Here's how the part is built. I have some questions about the finished solid (model axes, mm). Face numbers are marked on the shaded views. A direction names the side the tool comes from. Round coordinates to 2 decimals unless told otherwise and drop trailing zeros. Order: outer loops, then holes, each group sorted by start corner. A loop starts at its lowest first (then second) coordinate and runs counter-clockwise, first axis right, second up. Notation, with made-up numbers: (-25.75, -36) -> (-8.75, -36) arc R11 ccw to (-8.75, -18) -> close; hole circle Ø5 at (34, -5.5). An arc over 180 degrees is marked (long way). One line per item, written item: value.
```python
from build123d import *

# Parameters (mm, degrees)
F0_W     = 15
F0_H     = 20
F1_DEPTH = 17
F2_R     = 1.75
F3_DEPTH = 17.001
F2_W     = 15
F2_H     = 15
F4_DEPTH = 10
F5_R     = 1


with BuildPart() as f1:
    # F0 (on Top) → F1 (new body)
    with BuildSketch(Plane.XY):
        with Locations((-7.5, 10)):
            Rectangle(F0_W, F0_H)
    extrude(amount=F1_DEPTH)

    # F2 (on face) → F3 (cut, through all)
    with BuildSketch(Plane.XY.offset(17)):
        with Locations((-7.5, 10)):
            Circle(F2_R)
    extrude(amount=-F3_DEPTH, mode=Mode.SUBTRACT)

    # F2 (on face) → F4 (cut)
    with BuildSketch(Plane.XY.offset(17)):
        with Locations((-7.5, 7.5)):
            Rectangle(F2_W, F2_H)
        with Locations((-7.5, 10)):
            Circle(F2_R, mode=Mode.SUBTRACT)
    extrude(amount=-F4_DEPTH, mode=Mode.SUBTRACT)

    # F5
    f5_edges = [f1.edges().sort_by_distance(p)[0] for p in [
        (-7.5, 20, 17),
        (-7.5, 15, 17),
        (-7.5, 15, 7),
        (-7.5, 0, 7),
        (-15, 7.5, 7),
        (-15, 0, 3.5),
        (0, 15, 12),
        (0, 0, 3.5),
        (0, 17.5, 17),
        (-15, 17.5, 17),
        (0, 7.5, 7),
        (-15, 15, 12),
    ]]
    fillet(f5_edges, radius=F5_R)


solid = f1.part
```
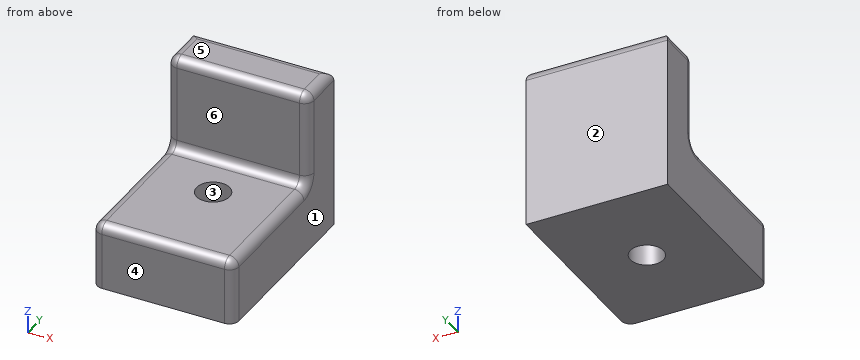
Q1. I need wall thicknesses on line 1 along Y through (x, z) = (-7.5, 5.5); line 2 along Z through (x, y) = (-6.25, 1.75); line 3 along Y through (x, z) = (-7.75, 13). Which ranges of each line are inside material? Lowest first, please.
Answers:
line 1: 0 to 8.25, 11.75 to 20
line 2: 0 to 7
line 3: 15 to 20
Q2. I want a section at B-B on z = 2. Write out the boundary of the cut face in (x, y).
Answers:
outline: (-15, 1) arc R1 ccw to (-14, 0) -> (-1, 0) arc R1 ccw to (0, 1) -> (0, 20) -> (-15, 20) -> close; hole circle Ø3.5 at (-7.5, 10)
Q3. Which directions (+Z, -Z, +X, -X, +Y, -Y) give clear straight access to the entire face, cutting with the end or side of a thin tool? Please do the marked faces 5 and 6.
Answers:
face 5: +Z, +X, -X, +Y, -Y
face 6: +Z, +X, -X, -Y
Q4. I want a section at C-C on x = -7.5. Write out the boundary of the cut face in (y, z), then the cut area to 3 significant figures.
Answers:
outline: (0, 0) -> (8.25, 0) -> (8.25, 7) -> (1, 7) arc R1 ccw to (0, 6) -> close; (11.75, 0) -> (20, 0) -> (20, 16) arc R1 ccw to (19, 17) -> (16, 17) arc R1 ccw to (15, 16) -> (15, 8) arc R1 cw to (14, 7) -> (11.75, 7) -> close
area: 165 mm2
Q5. If we mould it in two halves opening along Y, with no side actions, what happens to the marked faces 1, 2, 3 and 4? For each: pulls with the +Y half, pulls with the -Y half, needs draft (parallel to the pull), parting line crosses it, or undercut.
Answers:
face 1: needs draft
face 2: pulls with the +Y half
face 3: undercut
face 4: pulls with the -Y half
Q6. I want a section at A-A on y = 10. Write out the boundary of the cut face in (x, z), then the cut area to 3 significant figures.
Answers:
outline: (-15, 0) -> (-9.25, 0) -> (-9.25, 7) -> (-14, 7) arc R1 ccw to (-15, 6) -> close; (-5.75, 0) -> (0, 0) -> (0, 6) arc R1 ccw to (-1, 7) -> (-5.75, 7) -> close
area: 80.1 mm2
Q7. I want a section at D-D on z = 13.25. Write out the boundary of the cut face in (x, y).
Answers:
outline: (-15, 16) arc R1 ccw to (-14, 15) -> (-1, 15) arc R1 ccw to (0, 16) -> (0, 20) -> (-15, 20) -> close
Q8. For P1, Ø2, axis at y = 4, z = 9.5, coming from the +X side; P2, Ø4, axis at x = -6.5, y = 6.5, coming from the +Z side; P3, Ø9, axis at x = -5, z = 13.5, coming from the -Y side, each with a flat end and sliding along its axis, tell me the tip position at first contact or that it passes through.
Answers:
P1: through
P2: z = 7
P3: y = 15
